Here's how the part is built. I have some questions about the finished solid (model axes, mm). Face numbers are marked on the shaded views. A direction names the side the tool comes from. Coordinates: 2 decimals unless noted, no trailing zeros. Write each loop counter-clockwise with the first axis right and the second up, starting at its lowest first coordinate (ties: lowest second). Pieces come first, ordered by that corner, then holes. Notation, with made-up numbers: M -27.5,78.25 L 21.5,78.25 A20 ccw 21.5,117.25 Z; hole C -40,-10 d6. An arc over 180 degrees is marked long. Use a Markdown table: item, result.
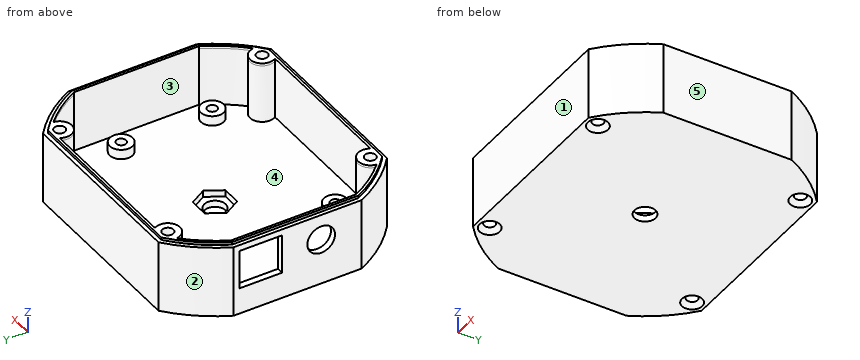
```python
from build123d import *

# Parameters (mm, degrees)
F0_R      = 1.7
F1_DEPTH  = 22
F2_T      = -2
F3_SIZE   = 1.4
F4_R      = 1.7
F5_DEPTH  = 0.8
F6_R      = 3.5
F6_R_2    = 1.5
F7_DEPTH  = 5
F8_W      = 13
F8_H      = 12
F8_R      = 4.25
F9_DEPTH  = 2
F10_R     = 3.5
F11_DEPTH = 2
F12_D     = 6.5


# Not quite as in the source:
# - a feature names something its author has since deleted; it is built from what else it names


with BuildPart() as f1:
    # F0 (on Top) → F1 (new body)
    with BuildSketch(Plane.XY):
        with BuildLine():
            Line((-40.5, 19.6150452459), (-40.5, -19.6150452459))
            ThreePointArc((-40.5, -19.6150452459), (-35.2419239111, -27.982258648), (-28.2842712475, -35))
            Line((-28.2842712475, -35), (28.2842712475, -35))
            ThreePointArc((28.2842712475, -35), (35.2419239111, -27.982258648), (40.5, -19.6150452459))
            Line((40.5, -19.6150452459), (40.5, 19.6150452459))
            ThreePointArc((40.5, 19.6150452459), (35.2419239111, 27.982258648), (28.2842712475, 35))
            Line((28.2842712475, 35), (-28.2842712475, 35))
            ThreePointArc((-28.2842712475, 35), (-35.2419239111, 27.982258648), (-40.5, 19.6150452459))
        make_face()
        with Locations((-26.5, -31)):
            Circle(F0_R, mode=Mode.SUBTRACT)
        with Locations((26.5, -31)):
            Circle(F0_R, mode=Mode.SUBTRACT)
        with Locations((-26.5, 31)):
            Circle(F0_R, mode=Mode.SUBTRACT)
        with Locations((26.5, 31)):
            Circle(F0_R, mode=Mode.SUBTRACT)
    extrude(amount=F1_DEPTH)

    # F2
    f2_openings = [f1.faces().sort_by_distance(p)[0] for p in [
        (0, 0, 22),
    ]]
    offset(amount=F2_T, openings=f2_openings)

    # F3
    f3_edges = [f1.edges().sort_by_distance(p)[0] for p in [
        (-28.2, -31, 0),
        (24.8, -31, 0),
        (24.8, 31, 0),
        (-28.2, 31, 0),
    ]]
    chamfer(f3_edges, length=F3_SIZE)

    # F4 (on face) → F5 (join)
    with BuildSketch(Plane.XY.offset(22)):
        with BuildLine():
            Line((27.8567765544, 33.8), (-27.8567765544, 33.8))
            ThreePointArc((-27.8567765544, 33.8), (-34.3481740656, 27.1779862823), (-39.3, 19.3377868434))
            Line((-39.3, 19.3377868434), (-39.3, -19.3377868434))
            ThreePointArc((-39.3, -19.3377868434), (-34.3481740656, -27.1779862823), (-27.8567765544, -33.8))
            Line((-27.8567765544, -33.8), (27.8567765544, -33.8))
            ThreePointArc((27.8567765544, -33.8), (34.3481740656, -27.1779862823), (39.3, -19.3377868434))
            Line((39.3, -19.3377868434), (39.3, 19.3377868434))
            ThreePointArc((39.3, 19.3377868434), (34.3481740656, 27.1779862823), (27.8567765544, 33.8))
        make_face()
        with Locations((-26.5, -31)):
            Circle(F4_R, mode=Mode.SUBTRACT)
        with Locations((26.5, -31)):
            Circle(F4_R, mode=Mode.SUBTRACT)
        with Locations((-26.5, 31)):
            Circle(F4_R, mode=Mode.SUBTRACT)
        with BuildLine():
            ThreePointArc((30.1812784263, -30.6282619904), (25.2805511537, -27.5067286806), (23.3871235167, -33))
            Line((23.3871235167, -33), (-23.3871235167, -33))
            ThreePointArc((-23.3871235167, -33), (-22.949813879, -32.0421988802), (-22.8, -31))
            ThreePointArc((-22.8, -31), (-26.3138954292, -27.3046833574), (-30.1812784263, -30.6282619904))
            ThreePointArc((-30.1812784263, -30.6282619904), (-34.8168494492, -25.2346387815), (-38.5, -19.1507180022))
            Line((-38.5, -19.1507180022), (-38.5, 19.1507180022))
            ThreePointArc((-38.5, 19.1507180022), (-34.8168494492, 25.2346387815), (-30.1812784263, 30.6282619904))
            ThreePointArc((-30.1812784263, 30.6282619904), (-26.3138954292, 27.3046833574), (-22.8, 31))
            ThreePointArc((-22.8, 31), (-22.949813879, 32.0421988802), (-23.3871235167, 33))
            Line((-23.3871235167, 33), (23.3871235167, 33))
            ThreePointArc((23.3871235167, 33), (25.2805511537, 27.5067286806), (30.1812784263, 30.6282619904))
            ThreePointArc((30.1812784263, 30.6282619904), (34.8168494492, 25.2346387815), (38.5, 19.1507180022))
            Line((38.5, 19.1507180022), (38.5, -19.1507180022))
            ThreePointArc((38.5, -19.1507180022), (34.8168494492, -25.2346387815), (30.1812784263, -30.6282619904))
        make_face(mode=Mode.SUBTRACT)
        with Locations((26.5, 31)):
            Circle(F4_R, mode=Mode.SUBTRACT)
    extrude(amount=F5_DEPTH)

    # F6 (on face) → F7 (join)
    with BuildSketch(Plane.XY.offset(2)):
        with Locations((-19, 24.05)):
            Circle(F6_R)
        with Locations((-19, 24.05)):
            Circle(F6_R_2, mode=Mode.SUBTRACT)
        with Locations((31.8, 8.85)):
            Circle(F6_R)
        with Locations((31.8, 8.85)):
            Circle(F6_R_2, mode=Mode.SUBTRACT)
        with Locations((31.8, -19.05)):
            Circle(F6_R)
        with Locations((31.8, -19.05)):
            Circle(F6_R_2, mode=Mode.SUBTRACT)
        with Locations((-20.3, -24.15)):
            Circle(F6_R)
        with Locations((-20.3, -24.15)):
            Circle(F6_R_2, mode=Mode.SUBTRACT)
    extrude(amount=F7_DEPTH)

    # F8 (on face) → F9 (cut, through all)
    with BuildSketch(Plane(origin=(-40.5, 0, 0), x_dir=(0, -1, 0), z_dir=(-1, 0, 0))):
        with Locations((-11.3, 14.1)):
            Rectangle(F8_W, F8_H)
        with Locations((7.2, 14.1)):
            Circle(F8_R)
    extrude(amount=-F9_DEPTH, mode=Mode.SUBTRACT)

    # F10 (on face) → F11 (join)
    with BuildSketch(Plane.XY.offset(2)):
        with BuildLine():
            ThreePointArc((-23.3871235167, 33), (-25.2805511537, 27.5067286806), (-30.1812784263, 30.6282619904))
            ThreePointArc((-30.1812784263, 30.6282619904), (-34.8168494492, 25.2346387815), (-38.5, 19.1507180022))
            Line((-38.5, 19.1507180022), (-38.5, -19.1507180022))
            ThreePointArc((-38.5, -19.1507180022), (-34.8168494492, -25.2346387815), (-30.1812784263, -30.6282619904))
            ThreePointArc((-30.1812784263, -30.6282619904), (-25.2805511537, -27.5067286806), (-23.3871235167, -33))
            Line((-23.3871235167, -33), (23.3871235167, -33))
            ThreePointArc((23.3871235167, -33), (25.2805511537, -27.5067286806), (30.1812784263, -30.6282619904))
            ThreePointArc((30.1812784263, -30.6282619904), (34.8168494492, -25.2346387815), (38.5, -19.1507180022))
            Line((38.5, -19.1507180022), (38.5, 19.1507180022))
            ThreePointArc((38.5, 19.1507180022), (34.8168494492, 25.2346387815), (30.1812784263, 30.6282619904))
            ThreePointArc((30.1812784263, 30.6282619904), (25.2805511537, 27.5067286806), (23.3871235167, 33))
            Line((23.3871235167, 33), (-23.3871235167, 33))
        make_face()
        with Locations((-20.3, -24.15)):
            Circle(F10_R, mode=Mode.SUBTRACT)
        with Locations((31.8, -19.05)):
            Circle(F10_R, mode=Mode.SUBTRACT)
        with Locations((-19, 24.05)):
            Circle(F10_R, mode=Mode.SUBTRACT)
        Polygon((-5.7735026919, 0), (-2.8867513459, 5), (2.8867513459, 5), (5.7735026919, 0), (2.8867513459, -5), (-2.8867513459, -5), align=None, mode=Mode.SUBTRACT)
        with Locations((31.8, 8.85)):
            Circle(F10_R, mode=Mode.SUBTRACT)
    extrude(amount=F11_DEPTH)

    # F12 (through all)
    with Locations(Plane.XY.offset(2)):
        with Locations((0, 0)):
            Hole(F12_D / 2)


solid = f1.part
```
1. Suppose I cut it at B-B on y = -9. Write out the boundary of the cut face in (x, z).
Answers follow:
| item | result |
|---|---|
| outline | M -40.5,0 L 40.5,0 L 40.5,22 L 39.3,22 L 39.3,22.8 L 38.5,22.8 L 38.5,4 L -38.5,4 L -38.5,10.25 L -40.5,10.25 Z; M -40.5,17.95 L -38.5,17.95 L -38.5,22.8 L -39.3,22.8 L -39.3,22 L -40.5,22 Z |
2. Suppose I cut it at D-D on z = 12.5. State how many separate pieces and enclosed holes the cut face has, and give its area (3 significant figures).
Answers follow:
| item | result |
|---|---|
| separate pieces | 2 |
| enclosed holes | 4 |
| area | 582 mm2 |
3. We'd pull the mould along X, two halves only. Please class the marked faces 1, 2 and 3: +X half, -X half, draft (parallel to the pull), parting line (faces both ways), or undercut.
Answers follow:
| item | result |
|---|---|
| face 1 | draft |
| face 2 | -X half |
| face 3 | undercut |
4. Suppose I cut it at A-A on x = 26.5. Write out the boundary of the cut face in (y, z).
Answers follow:
| item | result |
|---|---|
| outline | M -35,0 L -34.1,0 L -32.7,1.4 L -32.7,22.8 L -33.8,22.8 L -33.8,22 L -35,22 Z; M -29.3,1.4 L -27.9,0 L 27.9,0 L 29.3,1.4 L 29.3,22.8 L 27.3,22.8 L 27.3,4 L -27.3,4 L -27.3,22.8 L -29.3,22.8 Z; M 32.7,1.4 L 34.1,0 L 35,0 L 35,22 L 33.8,22 L 33.8,22.8 L 32.7,22.8 Z |
5. Which directions (+Z, -Z, +X, -X, +Y, -Y) give clear straight access to the entire face, cutting with the end or side of a thin tool? Please do the marked faces 4 and 5.
Answers follow:
| item | result |
|---|---|
| face 4 | +Z |
| face 5 | +Z, -Z, +X, +Y, -Y |
6. Will these pins go through, and if not, where does the flat tip stop? pin 1 Ø8 at (y, z) = (27, 2.5) entering from -X; pin 2 Ø1.8 at (x, y) = (-19, 24.05) entering from +Z; pin 3 Ø3.5 at (x, y) = (31.5, -19.5) entering from +Z; pin 4 Ø2 at (x, y) = (26.5, 31) entering from -Z.
Answers follow:
| item | result |
|---|---|
| pin 1 | stops at x = -38.68 |
| pin 2 | stops at z = 2 |
| pin 3 | stops at z = 7 |
| pin 4 | passes through |
7. Suppose I cut it at C-C on z = 21. Write out the boundary of the cut face in (x, y), and give its area (3 significant figures).
Answers follow:
| item | result |
|---|---|
| outline | M -40.5,-19.62 A45 ccw -28.28,-35 L 28.28,-35 A45 ccw 40.5,-19.62 L 40.5,19.62 A45 ccw 28.28,35 L -28.28,35 A45 ccw -40.5,19.62 Z; hole M -38.5,-19.15 A43 ccw -30.18,-30.63 A3.7 cw long -23.39,-33 L 23.39,-33 A3.7 cw long 30.18,-30.63 A43 ccw 38.5,-19.15 L 38.5,19.15 A43 ccw 30.18,30.63 A3.7 cw long 23.39,33 L -23.39,33 A3.7 cw long -30.18,30.63 A43 ccw -38.5,19.15 Z; hole C -26.5,-31 d3.4; hole C -26.5,31 d3.4; hole C 26.5,-31 d3.4; hole C 26.5,31 d3.4 |
| area | 624 mm2 |
8. I need wall thicknesses on probe 1 along Y at (x, z) = (26.5, 14.5); probe 2 along Y at (x, z) = (19, 21.5); probe 3 along Y at (x, z) = (0, 1.25). Which ranges of each line are inside material? Lowest first, please.
Answers follow:
| item | result |
|---|---|
| probe 1 | y = -35 to -32.7, -29.3 to -27.3, 27.3 to 29.3, 32.7 to 35 |
| probe 2 | y = -35 to -33, 33 to 35 |
| probe 3 | y = -35 to -3.25, 3.25 to 35 |
